from build123d import *

# Parameters (mm, degrees)
SKETCH_1_W      = 30
SKETCH_1_H      = 30
SKETCH_1_R      = 1.5
EXTRUDE_1_DEPTH = 4


with BuildPart() as part:
    # 草图1 → 凸台-拉伸1 (new body)
    with BuildSketch(Plane(origin=(0, 0, 0), x_dir=(1, 0, 0), z_dir=(0, 1, 0))):
        with Locations((15, -15)):
            Rectangle(SKETCH_1_W, SKETCH_1_H)
        with Locations(Location((8.5, -7, 0), (0, 0, 270))):
            Circle(SKETCH_1_R, mode=Mode.SUBTRACT)
        with Locations(Location((22.5, -7, 0), (0, 0, 270))):
            Circle(SKETCH_1_R, mode=Mode.SUBTRACT)
        with Locations(Location((22.5, -23, 0), (0, 0, 90))):
            Circle(SKETCH_1_R, mode=Mode.SUBTRACT)
        with Locations(Location((8.5, -23, 0), (0, 0, 90))):
            Circle(SKETCH_1_R, mode=Mode.SUBTRACT)
        Polygon((15, -12.5), (12.75, -16.5), (17.25, -16.5), align=None, mode=Mode.SUBTRACT)
    extrude(amount=EXTRUDE_1_DEPTH)


solid = part.part
The listing builds one solid part. Answer for the finished solid, in the listing's coordinates (mm). A direction names the side the tool comes from. Coordinates: 2 decimals unless noted, no trailing zeros. Loops run counter-clockwise (first coordinate to the right, second up) from the corner with the lowest first, then second, coordinate; pieces in that order, holes last.
1) Determine the mould class of faces 3 (the face through (15, 2, 16.5)), 4 (the face through (15, 2, 30)), 5 (the face through (30, 2, 15)) for opening direction X: pulls with the +X half, pulls with the -X half, needs draft (parallel to the pull), parting line crosses it, or undercut.
2) Find section C-C on y = 1.2. Write down the section's boundary in (x, z).
3) Find section A-A on z = 23. Write down the section's boundary in (x, y), then the cut area to 3 significant figures.
4) A tool of negligible diameter and unlimited length cuts with its end or side. For faces 1 (the face through (0, 2, 15)), 2 (the face through (13.89, 1.97, 14.47)), from which of +Z, -Z, +X, -X, +Y, -Y can it reach the whole face along a straight path? Write none if from no direction.
5) Find section B-B on x = 22.5. Write down the section's boundary in (y, z), then the cut area to 3 significant figures.
6) Find the intervals of material crossed by L1, parallel to X at y = 2.5, z = 23; L2, parallel to X at y = 0.75, z = 14.25; L3, parallel to X at y = 0.65, z = 13.75, in increasing order.
Values:
1. face 3: undercut
1. face 4: needs draft
1. face 5: pulls with the +X half
2. outline: (0, 0) - (30, 0) - (30, 30) - (0, 30) - close; hole circle Ø3 at (8.5, 7); hole circle Ø3 at (8.5, 23); hole (12.75, 16.5) - (15, 12.5) - (17.25, 16.5) - close; hole circle Ø3 at (22.5, 7); hole circle Ø3 at (22.5, 23)
3. outline: (0, 0) - (7, 0) - (7, 4) - (0, 4) - close; (10, 0) - (21, 0) - (21, 4) - (10, 4) - close; (24, 0) - (30, 0) - (30, 4) - (24, 4) - close
3. area: 96.0 mm2
4. face 1: +Z, -Z, -X, +Y, -Y
4. face 2: +Y, -Y
5. outline: (0, 0) - (4, 0) - (4, 5.5) - (0, 5.5) - close; (0, 8.5) - (4, 8.5) - (4, 21.5) - (0, 21.5) - close; (0, 24.5) - (4, 24.5) - (4, 30) - (0, 30) - close
5. area: 96.0 mm2
6. L1: x = 0 to 7, 10 to 21, 24 to 30
6. L2: x = 0 to 14.02, 15.98 to 30
6. L3: x = 0 to 14.3, 15.7 to 30
